Geometry: final body of the model. Coordinates: model frame, mm. Give positions to 0.01 mm unless a question says otherwise; leave off trailing zeros. Order: outer loops, then holes, each group sorted by start corner. A loop starts at its lowest first (then second) coordinate and runs counter-clockwise, first axis right, second up. Notation, with made-up numbers: (47.25, 9) - (60.25, 9) arc R13 ccw to (60.25, 27) - close; hole circle Ø11 at (-23.5, 28.5). An arc over 180 degrees is marked (long way). Use one line per item in the form item = value.
from build123d import *

# Parameters (mm, degrees)
SALIENTE_EXTRUIR1_DEPTH = 36.76416917
CORTAR_EXTRUIR1_REACH   = 46.527


with BuildPart() as part:
    # Croquis1 → Saliente-Extruir1 (new body)
    with BuildSketch(Plane.XY):
        with BuildLine():
            Line((-24.95, 2.07), (-24.95, 5))
            Line((-24.95, 5), (-22.8, 5))
            ThreePointArc((-22.8, 5), (-22.55695313, 4.875864205), (-22.515045035, 4.606188125))
            Line((-22.515045035, 4.606188125), (-23.35, 2.07))
            Line((-23.35, 2.07), (-24.95, 2.07))
        make_face()
    extrude(amount=-SALIENTE_EXTRUIR1_DEPTH)

    # Cortar-Extruir1: up to this face of the body (flat: up to its plane)
    cortar_extruir1_end = Plane(part.part.faces().sort_by_distance((-24.15, 2.07, -18.382084585))[0])
    # Croquis3 → Cortar-Extruir1 (cut, up to the picked face)
    with BuildSketch(Plane(origin=(0, 5, 0), x_dir=(1, 0, 0), z_dir=(0, 1, 0)), mode=Mode.PRIVATE) as cortar_extruir1_sk1:
        with BuildLine():
            Line((-24.95, 36.76416917), (-22.792893219, 34.607062389))
            ThreePointArc((-22.792893219, 34.607062389), (-22.576120467, 34.28263904), (-22.5, 33.899955608))
            Line((-22.5, 33.899955608), (-22.5, 2.864213562))
            ThreePointArc((-22.5, 2.864213562), (-22.576120467, 2.48153013), (-22.792893219, 2.157106781))
            Line((-22.792893219, 2.157106781), (-24.95, 0))
            Line((-24.95, 0), (-24.95, -1.353882683))
            Line((-24.95, -1.353882683), (-20.676224188, -1.353882683))
            Line((-20.676224188, -1.353882683), (-20.676224188, 38.571872723))
            Line((-20.676224188, 38.571872723), (-24.95, 38.571872723))
            Line((-24.95, 38.571872723), (-24.95, 36.76416917))
        make_face()
    cortar_extruir1_tool1 = split(extrude(cortar_extruir1_sk1.sketch, amount=-CORTAR_EXTRUIR1_REACH, mode=Mode.PRIVATE), bisect_by=cortar_extruir1_end, keep=Keep.BOTH, mode=Mode.PRIVATE)
    add(cortar_extruir1_tool1.solids().sort_by(Axis((-21.899514, 5, -18.829145), (0, -1, 0)))[0], mode=Mode.SUBTRACT)


solid = part.part
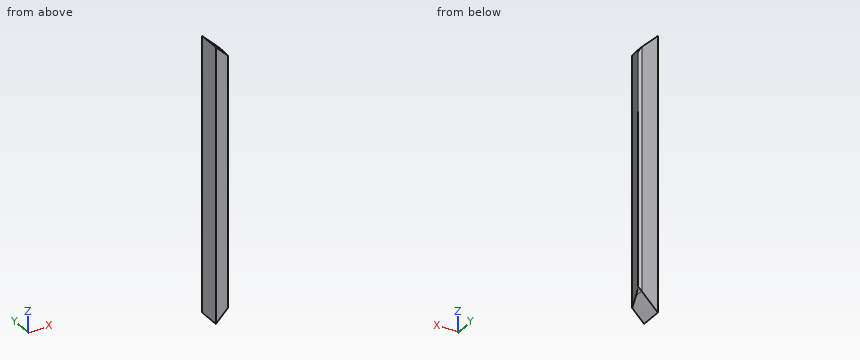
(1) Cut plane A-A on z = -12. Output: boundary loops of the cut face in (x, y), plus the area to 3 significant figures.
Computed values:
outline = (-24.95, 2.07) - (-23.35, 2.07) - (-22.52, 4.61) arc R0.3 ccw to (-22.8, 5) - (-24.95, 5) - close
area = 6.06 mm²
(2) Cut plane D-D on y = 2.4. Output: boundary loops of the cut face in (x, z).
Computed values:
outline = (-24.95, -36.76) - (-23.24, -35.06) - (-23.24, -1.71) - (-24.95, 0) - close
(3) Cut plane C-C on x = -23.95. Output: boundary loops of the cut face in (y, z), plus the area to 3 significant figures.
Computed values:
outline = (2.07, -35.76) - (5, -35.76) - (5, -1) - (2.07, -1) - close
area = 102 mm²
(4) Ray query, line 1 along X through (y, z) = (4.8, -20); line 2 along Z through (x, y) = (-23.35, 4.95); line 3 along X through (y, z) = (3.75, -12.5). Return the intervals inside material, ascending.
Computed values:
line_1 = -24.95 to -22.52
line_2 = -35.16 to -1.6
line_3 = -24.95 to -22.8
(5) Cut plane B-B on y = 4.1. Output: boundary loops of the cut face in (x, z), plus the area to 3 significant figures.
Computed values:
outline = (-24.95, -36.76) - (-22.79, -34.61) arc R1 ccw to (-22.68, -34.47) - (-22.68, -2.29) arc R1 ccw to (-22.79, -2.16) - (-24.95, 0) - close
area = 78.2 mm²
